Here's how the part is built. I have some questions about the finished solid (model axes, mm). A direction names the side the tool comes from. Round coordinates to 2 decimals unless told otherwise and drop trailing zeros. Order: outer loops, then holes, each group sorted by start corner. A loop starts at its lowest first (then second) coordinate and runs counter-clockwise, first axis right, second up.
```python
from build123d import *

# Parameters (mm, degrees)
SKETCH1_W           = 15
SKETCH1_H           = 7
SKETCH1_R           = 1.5
SKETCH1_R_2         = 1.715572335
BOSS_EXTRUDE1_DEPTH = 3
CHAMFER1_SIZE       = 10


with BuildPart() as part:
    # Sketch1 → Boss-Extrude1 (new body)
    # profile 1 of 5: a face of its own
    with BuildSketch(Plane.XY):
        Polygon((15, 162), (0, 162), (0, 0), (15, 0), (197, 0), (212, 0), (212, 162), (197, 162), align=None)
        Polygon((126, 151), (201, 151), (201, 11), (126, 11), (126, 63.5), (36, 63.5), (36, 98.5), (126, 98.5), align=None, mode=Mode.SUBTRACT)
    # profile 2 of 5: a face of its own
    with BuildSketch(Plane.XY):
        with Locations((7.5, 165.5)):
            Rectangle(SKETCH1_W, SKETCH1_H)
        with Locations((11, 165.5)):
            Circle(SKETCH1_R, mode=Mode.SUBTRACT)
    # profile 3 of 5: a face of its own
    with BuildSketch(Plane.XY):
        with Locations((7.5, -3.5)):
            Rectangle(SKETCH1_W, SKETCH1_H)
        with Locations((11, -3.5)):
            Circle(SKETCH1_R, mode=Mode.SUBTRACT)
    # profile 4 of 5: a face of its own
    with BuildSketch(Plane.XY):
        with Locations((204.5, -3.5)):
            Rectangle(SKETCH1_W, SKETCH1_H)
        with Locations((208, -3.5)):
            Circle(SKETCH1_R_2, mode=Mode.SUBTRACT)
    # profile 5 of 5: a face of its own
    with BuildSketch(Plane.XY):
        with Locations((204.5, 165.5)):
            Rectangle(SKETCH1_W, SKETCH1_H)
        with Locations((208, 165.5)):
            Circle(SKETCH1_R_2, mode=Mode.SUBTRACT)
    extrude(amount=BOSS_EXTRUDE1_DEPTH)

    # Chamfer1
    chamfer1_edges = [part.edges().sort_by_distance(p)[0] for p in [
        (126, 98.5, 1.5),
        (126, 63.5, 1.5),
    ]]
    chamfer(chamfer1_edges, length=CHAMFER1_SIZE)


solid = part.part
```
1) If we section it at D-D (x = 32.5): Write out the boundary of the cut face in (y, z), plus the area to 3 significant figures.
2) If we section it at C-C (y = 73.5): Write out the boundary of the cut face in (x, z).
3) I'm going to push flat-ended pins straight in: pin 1 (2.5 mm diameter, centred on x = 208, y = -3.5, fed in from +Z); pin 2 (1.5 mm diameter, centred on x = 182, z = 1.5, fed in from +Y); pin 3 (0.9 mm diameter, centred on x = 139.5, z = 2, fed in from -Y). Where does each tip first touch, or does it pass through?
4) If we section it at B-B (z = 0.5): Write out the boundary of the cut face in (x, y), plus the area to 3 significant figures.
5) We'd pull the mould along X, two halves only. Please class faces 3 (the flat face through (120.9, 103.4, 1.5)), 4 (the flat face through (81, 63, 3)): +X half, -X half, draft (parallel to the pull), parting line (faces both ways), or undercut.
6) For faces 1 (the flat face through (121.1, 58.4, 1.5)), 2 (the flat face through (81, 63, 0)), which set-ups out of +Z, -Z, +X, -X, +Y, -Y let a thin tool reach every point of the face, with its end or its side?
7) If we section it at A-A (x = 123.5): Write out the boundary of the cut face in (y, z).
8) I need wall thicknesses on line 1 (Y direction, x = 208, z = 1.85); line 2 (Y direction, x = 11, z = 0.95); line 3 (X direction, y = 165.5, z = 1.5). Which ranges of each line are inside material? Lowest first, please.
Solutions:
1. outline: (0, 0) - (162, 0) - (162, 3) - (0, 3) - close
1. area: 486 mm2
2. outline: (0, 0) - (36, 0) - (36, 3) - (0, 3) - close; (201, 0) - (212, 0) - (212, 3) - (201, 3) - close
3. pin 1: passes through
3. pin 2: stops at y = 162
3. pin 3: stops at y = 0
4. outline: (0, -7) - (15, -7) - (15, 0) - (197, 0) - (197, -7) - (212, -7) - (212, 169) - (197, 169) - (197, 162) - (15, 162) - (15, 169) - (0, 169) - close; hole circle Ø3 at (11, -3.5); hole circle Ø3 at (11, 165.5); hole (36, 63.5) - (116, 63.5) - (126, 53.5) - (126, 11) - (201, 11) - (201, 151) - (126, 151) - (126, 108.5) - (116, 98.5) - (36, 98.5) - close; hole circle Ø3.43 at (208, -3.5); hole circle Ø3.43 at (208, 165.5)
4. area: 21,000 mm2
5. face 3: undercut
5. face 4: draft
6. face 1: +Z, -Z
6. face 2: -Z, +X, -X, +Y, -Y
7. outline: (0, 0) - (56, 0) - (56, 3) - (0, 3) - close; (106, 0) - (162, 0) - (162, 3) - (106, 3) - close
8. line 1: y = -7 to -5.22, -1.78 to 163.78, 167.22 to 169
8. line 2: y = -7 to -5, -2 to 164, 167 to 169
8. line 3: x = 0 to 9.5, 12.5 to 15, 197 to 206.28, 209.72 to 212
